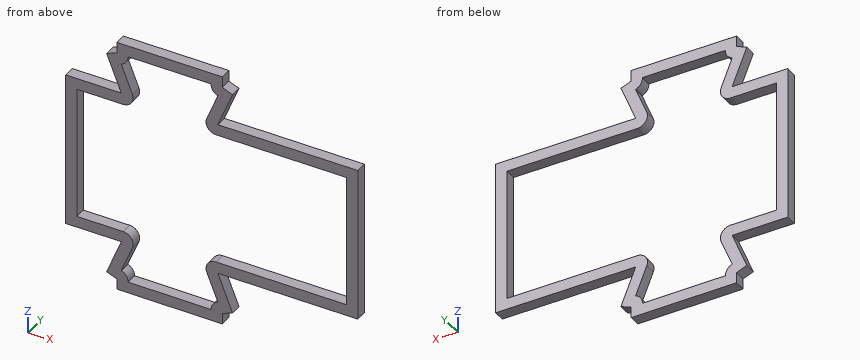
```python
from build123d import *

# Parameters (mm, degrees)
BOSS_EXTRUDE2_DEPTH = 10
FILLET2_R           = 9


with BuildPart() as part:
    # Sketch2 → Boss-Extrude2 (new body)
    with BuildSketch(Plane(origin=(0, 0, 0), x_dir=(1, 0, 0), z_dir=(0, 1, 0))):
        Polygon((-92.4, -69.4), (-92.4, 69.4), (-42.892169593, 69.4), (-55.995137589, 101.931506748), (-46.9, 105.594826054), (-46.9, 115.030994267), (46.9, 115.39765007), (46.9, 105.594826054), (55.995137589, 101.931506748), (42.892169593, 69.4), (167.4, 69.4), (167.4, -69.4), (42.892169593, -69.4), (55.995137589, -101.931506748), (46.9, -105.594826054), (46.9, -115.4), (-46.9, -115.4), (-46.9, -105.594826054), (-55.995137589, -101.931506748), (-42.892169593, -69.4), align=None)
        Polygon((-82.4, -59.4), (-82.4, 59.4), (-28.083714943, 59.4), (-42.983173736, 96.391759761), (-36.9, 98.84192696), (-36.9, 105.070006974), (36.9, 105.358484567), (36.9, 98.84192696), (42.983173736, 96.391759761), (28.083714943, 59.4), (157.4, 59.4), (157.4, -59.4), (28.083714943, -59.4), (42.983173736, -96.391759761), (36.9, -98.84192696), (36.9, -105.4), (-36.9, -105.4), (-36.9, -98.84192696), (-42.983173736, -96.391759761), (-28.083714943, -59.4), align=None, mode=Mode.SUBTRACT)
    extrude(amount=BOSS_EXTRUDE2_DEPTH)

    # Fillet2
    fillet2_edges = [part.edges().sort_by_distance(p)[0] for p in [
        (-28.083714943, 5, 59.4),
        (-36.9, 5, 98.84192696),
        (36.9, 5, 98.84192696),
        (28.083714943, 5, 59.4),
        (28.083714943, 5, -59.4),
        (36.9, 5, -98.84192696),
        (-36.9, 5, -98.84192696),
        (-28.083714943, 5, -59.4),
    ]]
    fillet(fillet2_edges, radius=FILLET2_R)


solid = part.part
```
Could you check a few things on this model? Use its own coordinates, in mm. Coordinates: 2 decimals unless noted, no trailing zeros. Write each loop counter-clockwise with the first axis right and the second up, starting at its lowest first coordinate (ties: lowest second). Pieces come first, ordered by that corner, then holes. Notation, with made-up numbers: (20.25, -35) -> (55.25, -35) arc R10 ccw to (55.25, -27) -> close; hole circle Ø11 at (39.25, -29). An arc over 180 degrees is marked (long way). Return JSON: item names as keys, results as strings.
(1) I'm going to push flat-ended pins straight in: pin 1 (5 mm diameter, centred on x = 97.5, y = 5.5, fed in from +Z); pin 2 (3 mm diameter, centred on y = 4.5, z = -111.5, fed in from -X); pin 3 (3 mm diameter, centred on x = -77.5, y = 5.5, fed in from -Z). Where does each tip first touch, or does it pass through?
Numbers:
{"pin 1": "stops at z = 69.4", "pin 2": "stops at x = -46.9", "pin 3": "stops at z = -69.4"}
(2) Imagine slicing it at B-B, the plane x = -12.5. Please give me the cut outline in (y, z), then the cut area to 3 significant figures.
Numbers:
{"outline": "(0, -115.17) -> (10, -115.17) -> (10, -105.17) -> (0, -105.17) -> close; (0, 105.4) -> (10, 105.4) -> (10, 115.4) -> (0, 115.4) -> close", "area": "200 mm2"}
(3) Imagine slicing it at A-A, the plane z = 38. Please give me the cut outline in (x, y), then the cut area to 3 significant figures.
Numbers:
{"outline": "(-92.4, 0) -> (-82.4, 0) -> (-82.4, 10) -> (-92.4, 10) -> close; (157.4, 0) -> (167.4, 0) -> (167.4, 10) -> (157.4, 10) -> close", "area": "200 mm2"}
(4) I need wall thicknesses on L1, parallel to Z at x = 102, y = 3; L2, parallel to X at y = 5.25, z = 20.5; L3, parallel to Z at x = 39.5, y = 8.5. Which ranges of each line are inside material? Lowest first, please.
Numbers:
{"L1": "z = -69.4 to -59.4, 59.4 to 69.4", "L2": "x = -92.4 to -82.4, 157.4 to 167.4", "L3": "z = -115.37 to -98.59, -87.74 to -59.61, 59.61 to 87.74, 98.59 to 115.4"}
